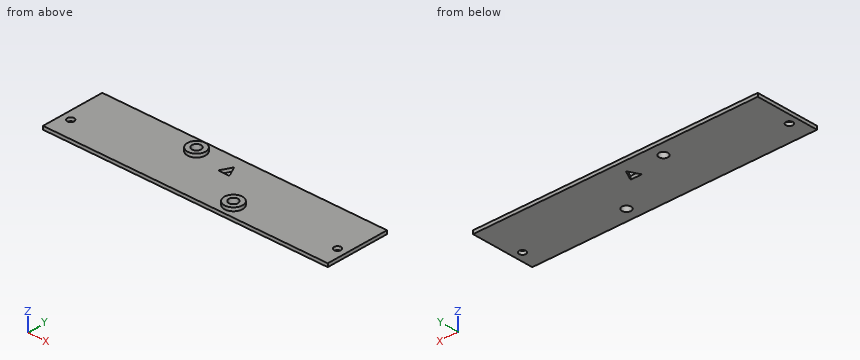
Autodesk Fusion 360 part; units mm, degrees
sketch "Sketch1" plane through (0, 0, 0) normal (0, 0, 1) x (1, 0, 0)
  line L0 (0, 0) -> (127.5, 0)
  line L1 (127.5, 0) -> (127.5, 28.5)
  line L2 (127.5, 28.5) -> (0, 28.5)
  line L3 (0, 28.5) -> (0, 0)
  circle A0 centre (4, 9) radius 1.55
  line L4 (63.75, 0) -> (63.75, 28.5) construction
  circle A1 centre (123.5, 9) radius 1.55
  line L5 (66.25, 18.5) -> (61.25, 18.5)
  line L6 (61.25, 18.5) -> (61.25, 23.5)
  line L7 (61.25, 23.5) -> (66.25, 23.5)
  line L8 (66.25, 23.5) -> (66.25, 18.5)
  line L9 (66.25, 18.5) -> (61.25, 23.5) construction
  line L10 (61.25, 18.5) -> (66.25, 23.5) construction
  line L11 (61.25, 18.5) -> (63.75, 23.5)
  line L12 (66.25, 18.5) -> (63.75, 23.5)
  point P0 (63.75, 21)
  dimension "d1" = 127.5
  dimension "d2" = 28.5
  dimension "d3" = 3.1
  dimension "d4" = 9
  dimension "d5" = 4
  dimension "d11" = 5
  dimension "d12" = 5
  dimension "d13" = 5
extrude "Extrude1" add sketch "Sketch1" along normal blind 1.5 contours L0 L1 L2 L3 | L7 L8 L12 | L6 L7 L11
sketch "Sketch2" plane through (0, 0, 1.5) normal (0, 0, 1) x (-1, 0, 0)
  circle A0 centre (-123.5, -9) radius 1.55
  circle A1 centre (-4, -9) radius 1.55
  line L0 (-66.25, -18.5) -> (-61.25, -18.5)
  line L1 (-61.25, -18.5) -> (-63.75, -23.5)
  line L2 (-63.75, -23.5) -> (-66.25, -18.5)
  line L3 (0, -28.5) -> (0, 0)
  line L4 (0, 0) -> (-127.5, 0)
  line L5 (-127.5, 0) -> (-127.5, -28.5)
  line L6 (-127.5, -28.5) -> (0, -28.5)
  line L7 (-63.75, -28.5) -> (-63.75, 0) construction
  line L8 (-87.75, -2.75) -> (-39.75, -2.75)
  line L9 (-39.75, -2.75) -> (-39.75, -25.75)
  line L10 (-39.75, -25.75) -> (-87.75, -25.75)
  line L11 (-87.75, -25.75) -> (-87.75, -2.75)
  line L12 (-87.75, -2.75) -> (-39.75, -25.75) construction
  line L13 (-39.75, -2.75) -> (-87.75, -25.75) construction
  circle A2 centre (-47.75, -22.55) radius 2.05
  circle A3 centre (-47.75, -22.55) radius 4.05
  circle A4 centre (-79.75, -5.95) radius 2.05
  circle A5 centre (-79.75, -5.95) radius 4.05
  point P0 (-63.75, -14.25)
  dimension "d14" = 48
  dimension "d15" = 23
  dimension "d18" = 8
  dimension "d19" = 3.2
  dimension "d20" = 4.1
  dimension "d21" = 8.1
  dimension "d22" = 4.1
  dimension "d23" = 8.1
  dimension "d24" = 8
  dimension "d25" = 3.2
extrude "Extrude2" add sketch "Sketch2" along normal blind 1.5 contours L8 A5 | L8 A5 | L10 A3 | L10 A3
extrude "Extrude3" cut sketch "Sketch2" against normal blind 1.5 contours A2 | A4
equation "d1 = 134 mm - 6 mm - 0.5 mm"
equation "d4 = 10.5 mm - 1.5 mm"
equation "d5 = 7 mm - 3 mm"
equation "d21 = d20 + 4 mm"
equation "d22 = d20"
equation "d23 = d21"
Here's how the part is built. I have some questions about the finished solid (model axes, mm). Give positions to 0.01 mm unless a question says otherwise; leave off trailing zeros. Order: outer loops, then holes, each group sorted by start corner. A loop starts at its lowest first (then second) coordinate and runs counter-clockwise, first axis right, second up. Notation, with made-up numbers: (46.25, 42) -> (90.25, 42) arc R10 ccw to (90.25, 47) -> close; hole circle Ø7 at (51, -34.5). An arc over 180 degrees is marked (long way). Use a Markdown table: item, result. Add a question column.
Item 1: Imagine slicing it at D-D on x = 15. Please give me the cut outline in (y, z), plus the area to 4 significant figures.
Item 2: Imagine slicing it at B-B on y = 5.95. Please give me the cut outline in (x, z), plus the area to 3 significant figures.
Item 3: Imagine slicing it at C-C on x = 123.5. Please give me the cut outline in (y, z).
Item 4: Imagine slicing it at A-A on x = 79.75. Please give me the cut outline in (y, z).
Item 5: I need wall thicknesses on line 1 (Y direction, x = 4, z = 0.65); line 2 (X direction, y = 9.5, z = 1.2); line 3 (X direction, y = 21.5, z = 1.3). Which ranges of each line are inside material? Lowest first, please.
Item 6: Will this pin go through, and if not, where does the flat tip stop? pin 1 (6 mm diameter, centred on x = 40, y = 22, fed in from +Z).
Data:
| question | item | result |
|---|---|---|
| 1 | outline | (0, 0) -> (28.5, 0) -> (28.5, 1.5) -> (0, 1.5) -> close |
| 1 | area | 42.75 mm² |
| 2 | outline | (0, 0) -> (77.7, 0) -> (77.7, 3) -> (75.7, 3) -> (75.7, 1.5) -> (0, 1.5) -> close; (81.8, 0) -> (127.5, 0) -> (127.5, 1.5) -> (83.8, 1.5) -> (83.8, 3) -> (81.8, 3) -> close |
| 2 | area | 191 mm² |
| 3 | outline | (0, 0) -> (7.45, 0) -> (7.45, 1.5) -> (0, 1.5) -> close; (10.55, 0) -> (28.5, 0) -> (28.5, 1.5) -> (10.55, 1.5) -> close |
| 4 | outline | (0, 0) -> (3.9, 0) -> (3.9, 3) -> (1.9, 3) -> (1.9, 1.5) -> (0, 1.5) -> close; (8, 0) -> (28.5, 0) -> (28.5, 1.5) -> (10, 1.5) -> (10, 3) -> (8, 3) -> close |
| 5 | line 1 | y = 0 to 7.45, 10.55 to 28.5 |
| 5 | line 2 | x = 0 to 2.53, 5.47 to 122.03, 124.97 to 127.5 |
| 5 | line 3 | x = 0 to 45.99, 49.51 to 62.75, 64.75 to 127.5 |
| 6 | pin 1 | stops at z = 1.5 |
